The model under review builds one solid part; all positions refer to its coordinate system, in mm. Face numbers are marked on the shaded views. A direction names the side the tool comes from. Round coordinates to 2 decimals unless told otherwise and drop trailing zeros. Order: outer loops, then holes, each group sorted by start corner. A loop starts at its lowest first (then second) coordinate and runs counter-clockwise, first axis right, second up. Notation, with made-up numbers: M 2.5,62.25 L 15.5,62.25 A18 cw 15.5,87.25 Z; hole C 39,47.25 d8. An arc over 180 degrees is marked long. Use a Markdown table: item, result. Add a question column.
1. Consider section A-A on x = 0. State the section outline as (y, z) points.
2. To check wall thickness, follow probe 1 along Y at (x, z) = (0.5, -16); probe 2 along Y at (x, z) = (37, -10); probe 3 along X at (y, z) = (35.5, 0.5). State the ranges of each line that lie inside material, in increasing order.
3. Consider section C-C on y = 26. State the section outline as (x, z) points, then the cut area to 3 significant figures.
4. Consider section B-B on z = 0. State the section outline as (x, y) points.
5. Insertion check: P1, Ø4, axis at y = -32, z = 2.5, coming from the +X side; P2, Ø4, axis at x = 22.5, z = 16, coming from the +Y side; P3, Ø8, axis at x = 7.5, y = -118.5, coming from the -Z side. Each pin has a flat end and moves straight along its axis. Give the tip position at first contact, or say it passes through.
6. For the marked faces 1, 2 and 3, list the 3-axis set-ups (+Z, -Z, +X, -X, +Y, -Y) from which the entire face can be reached by the end or side of a thin tool; tool diameter is ignored.
7. Consider section D-D on z = -19.5. State the section outline as (x, y) points.
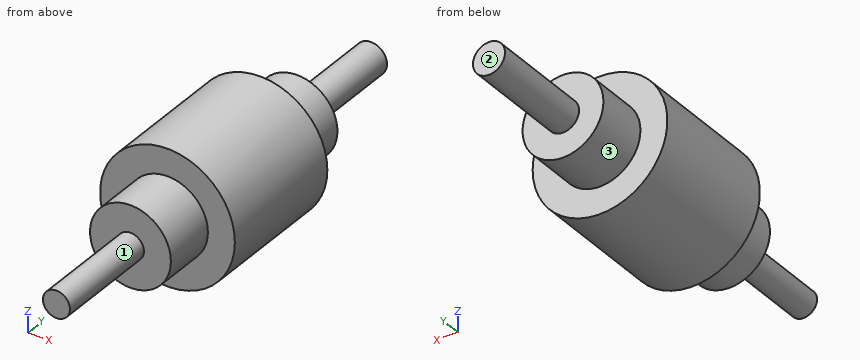
from build123d import *

# Parameters (mm, degrees)
F0_R      = 50
F1_DEPTH  = 40
F1_FACE_R = 50
F2_DEPTH  = 60
F3_R      = 30
F4_DEPTH  = 40
F5_R      = 10
F6_DEPTH  = 80
F7_R      = 30
F8_DEPTH  = 40
F9_R      = 11.8892
F10_DEPTH = 80


with BuildPart() as f1:
    # F0 (on Front) → F1 (new body)
    with BuildSketch(Plane.XZ):
        Circle(F0_R)
    extrude(amount=F1_DEPTH)

    # F1_face (on face) → F2 (join)
    with BuildSketch(Plane.XZ.offset(40)):
        Circle(F1_FACE_R)
    extrude(amount=F2_DEPTH)

    # F3 (on face) → F4 (join)
    with BuildSketch(Plane.XZ.offset(100)):
        Circle(F3_R)
    extrude(amount=F4_DEPTH)

    # F5 (on face) → F6 (join)
    with BuildSketch(Plane.XZ.offset(140)):
        Circle(F5_R)
    extrude(amount=F6_DEPTH)

    # F7 (on face) → F8 (join)
    with BuildSketch(Plane(origin=(0, 0, 0), x_dir=(-1, 0, 0), z_dir=(0, 1, 0))):
        Circle(F7_R)
    extrude(amount=F8_DEPTH)

    # F9 (on face) → F10 (join)
    with BuildSketch(Plane(origin=(0, 40, 0), x_dir=(-1, 0, 0), z_dir=(0, 1, 0))):
        Circle(F9_R)
    extrude(amount=F10_DEPTH)


solid = f1.part
Answer block:
| question | item | result |
|---|---|---|
| 1 | outline | M -220,-10 L -140,-10 L -140,-30 L -100,-30 L -100,-50 L 0,-50 L 0,-30 L 40,-30 L 40,-11.89 L 120,-11.89 L 120,11.89 L 40,11.89 L 40,30 L 0,30 L 0,50 L -100,50 L -100,30 L -140,30 L -140,10 L -220,10 Z |
| 2 | probe 1 | -140 to 40 |
| 2 | probe 2 | -100 to 0 |
| 2 | probe 3 | -30 to 30 |
| 3 | outline | C 0,0 d60 |
| 3 | area | 2,830 mm^2 |
| 4 | outline | M -50,-100 L -30,-100 L -30,-140 L -10,-140 L -10,-220 L 10,-220 L 10,-140 L 30,-140 L 30,-100 L 50,-100 L 50,0 L 30,0 L 30,40 L 11.89,40 L 11.89,120 L -11.89,120 L -11.89,40 L -30,40 L -30,0 L -50,0 Z |
| 5 | P1 | x = 50 |
| 5 | P2 | y = 40 |
| 5 | P3 | z = -29.8 |
| 6 | face 1 | -Y |
| 6 | face 2 | +Z, -Z, +X, -X, +Y |
| 6 | face 3 | +Y |
| 7 | outline | M -46.04,-100 L -22.8,-100 L -22.8,-140 L 22.8,-140 L 22.8,-100 L 46.04,-100 L 46.04,0 L 22.8,0 L 22.8,40 L -22.8,40 L -22.8,0 L -46.04,0 Z |
